Part model, mm, in its own coordinate system. A direction names the side the tool comes from. Give positions to 0.01 mm unless a question says otherwise; leave off trailing zeros. Order: outer loops, then holes, each group sorted by start corner. A loop starts at its lowest first (then second) coordinate and runs counter-clockwise, first axis right, second up. Notation, with made-up numbers: (29.5, 57.25) -> (86.5, 57.25) arc R20 ccw to (86.5, 94.25) -> close; hole circle Ø8 at (26.5, 24.25). An arc over 180 degrees is marked (long way). Write item = value, one per line. Start each with the question number.
Item 1: Band-saw the part on A-A on y = 3.5. Write the cut outline in (x, z), plus the area to 3 significant figures.
Item 2: Band-saw the part on C-C on y = -5. Write the cut outline in (x, z), plus the area to 3 significant figures.
Item 3: Tool access for faces 4 (the face through (8.3, 1, 1)), 5 (the face through (-4.1, -2.5, 0)): list every direction of +Z, -Z, +X, -X, +Y, -Y with a clear straight run to the whole face (end or side of a thin tool).
Item 4: Flat gauge pins, fed straight in: P1, Ø0.8, axis at x = 6.5, z = 1.5, coming from the -Y side; P2, Ø0.9, axis at y = 6.5, z = 2, coming from the -X side; P3, Ø1.5, axis at y = 7.5, z = 2, coming from the +X side. Where does each tip first touch, or does it go through?
Item 5: Band-saw the part on D-D on z = 1.1. Write the cut outline in (x, y), plus the area to 3 significant figures.
Item 6: Pull direction Y, two halves, no side cores. Call faces 1 (the face through (0, 10.5, 1)), 2 (the face through (-8.3, 1, 2)), 3 (the face through (-8.07, -9, 1.48)): +Y half, -Y half, draft (parallel to the pull), parting line (faces both ways), or undercut.
Item 7: Drill centre lines: line 1 along Y through (x, z) = (-5, 2.3); line 2 along Y through (x, z) = (-1.25, 0.5); line 3 along Y through (x, z) = (-4, 1.5). Where is each one in solid material? Low to high.
Item 8: Band-saw the part on B-B on x = 1.75. Write the cut outline in (y, z), plus the area to 3 significant figures.
```python
from build123d import *

# Parameters (mm, degrees)
RESSALTO_EXTRUS_O1_DEPTH = 3
CORTE_EXTRUS_O1_DEPTH    = 3
ESBO_O3_R                = 1.5
CORTE_EXTRUS_O2_DEPTH    = 3
CHANFRO1_SIZE            = 3
ESBO_O4_W                = 3
ESBO_O4_H                = 4
RESSALTO_EXTRUS_O2_DEPTH = 0.7
ESBO_O5_W                = 3
ESBO_O5_H                = 4
RESSALTO_EXTRUS_O3_DEPTH = 0.7


with BuildPart() as part:
    # Esboço1 → Ressalto-extrusão1 (new body)
    with BuildSketch(Plane.XY):
        with BuildLine():
            Line((4.5, 10.5), (-4.5, 10.5))
            ThreePointArc((-4.5, 10.5), (-8.035533906, 9.035533906), (-9.5, 5.5))
            Line((-9.5, 5.5), (-9.5, -5.5))
            ThreePointArc((-9.5, -5.5), (-8.035533906, -9.035533906), (-4.5, -10.5))
            Line((-4.5, -10.5), (4.5, -10.5))
            ThreePointArc((4.5, -10.5), (8.035533906, -9.035533906), (9.5, -5.5))
            Line((9.5, -5.5), (9.5, 5.5))
            ThreePointArc((9.5, 5.5), (8.035533906, 9.035533906), (4.5, 10.5))
        make_face()
    extrude(amount=RESSALTO_EXTRUS_O1_DEPTH)

    # Esboço2 → Corte-extrusão1 (cut)
    with BuildSketch(Plane(origin=(0, 0, 0), x_dir=(-1, 0, 0), z_dir=(0, 0, -1))):
        Polygon((-2.5, -1.5), (-2.5, -9), (1.5, -9), (1.5, -1.5), (9, -1.5), (9, 2.5), (1.5, 2.5), (1.5, 9), (-2.5, 9), (-2.5, 2.5), (-9, 2.5), (-9, -1.5), align=None)
    extrude(amount=-CORTE_EXTRUS_O1_DEPTH, mode=Mode.SUBTRACT)

    # Esboço3 → Corte-extrusão2 (cut)
    with BuildSketch(Plane.XY.offset(3)):
        with Locations((6, -5)):
            Circle(ESBO_O3_R)
        with Locations((-5, 6)):
            Circle(ESBO_O3_R)
    extrude(amount=-CORTE_EXTRUS_O2_DEPTH, mode=Mode.SUBTRACT)

    # Chanfro1
    chanfro1_edges = [part.edges().sort_by_distance(p)[0] for p in [
        (2.5, -1.5, 1.5),
        (2.5, 2.5, 1.5),
        (-1.5, 2.5, 1.5),
        (-1.5, -1.5, 1.5),
    ]]
    chamfer(chanfro1_edges, length=CHANFRO1_SIZE)

    # Esboço4 → Ressalto-extrusão2 (add)
    with BuildSketch(Plane(origin=(-9, 0, 0), x_dir=(0, 0, -1), z_dir=(1, 0, 0))):
        with Locations((-1.5, 0.5)):
            Rectangle(ESBO_O4_W, ESBO_O4_H)
    extrude(amount=RESSALTO_EXTRUS_O2_DEPTH)

    # Esboço5 → Ressalto-extrusão3 (add)
    with BuildSketch(Plane.ZY.offset(-9)):
        with Locations((1.5, 0.5)):
            Rectangle(ESBO_O5_W, ESBO_O5_H)
    extrude(amount=RESSALTO_EXTRUS_O3_DEPTH)


solid = part.part
```
Values found:
q1.outline = (-9.5, 0) -> (-3.5, 0) -> (-3.5, 3) -> (-9.5, 3) -> close; (4.5, 0) -> (9.5, 0) -> (9.5, 3) -> (4.5, 3) -> close
q1.area = 33.0 mm^2
q2.outline = (-9.5, 0) -> (-1.5, 0) -> (-1.5, 3) -> (-9.5, 3) -> close; (2.5, 0) -> (4.5, 0) -> (4.5, 3) -> (2.5, 3) -> close; (7.5, 0) -> (9.5, 0) -> (9.5, 3) -> (7.5, 3) -> close
q2.area = 36.0 mm^2
q3.face_4 = +Z, -Z
q3.face_5 = -Z, +X, -X, +Y, -Y
q4.P1 = -10.24
q4.P2 = -9.47
q4.P3 = 9.34
q5.outline = (-9.5, -5.5) arc R5 ccw to (-4.5, -10.5) -> (4.5, -10.5) arc R5 ccw to (9.5, -5.5) -> (9.5, 5.5) arc R5 ccw to (4.5, 10.5) -> (-4.5, 10.5) arc R5 ccw to (-9.5, 5.5) -> close; hole (-8.3, -1.5) -> (-4.5, -1.5) -> (-1.5, -4.5) -> (-1.5, -9) -> (2.5, -9) -> (2.5, -4.5) -> (5.5, -1.5) -> (8.3, -1.5) -> (8.3, 2.5) -> (5.5, 2.5) -> (2.5, 5.5) -> (2.5, 9) -> (-1.5, 9) -> (-1.5, 5.5) -> (-4.5, 2.5) -> (-8.3, 2.5) -> close; hole circle Ø3 at (-5, 6); hole circle Ø3 at (6, -5)
q5.area = 223 mm^2
q6.face_1 = +Y half
q6.face_2 = undercut
q6.face_3 = -Y half
q7.line_1 = -10.47 to -1.5, 2.5 to 4.5, 7.5 to 10.47
q7.line_2 = -10.5 to -9, 9 to 10.5
q7.line_3 = -10.5 to -2, 3 to 4.88, 7.12 to 10.5
q8.outline = (-10.5, 0) -> (-9, 0) -> (-9, 3) -> (-10.5, 3) -> close; (9, 0) -> (10.5, 0) -> (10.5, 3) -> (9, 3) -> close
q8.area = 9.00 mm^2
